Work out the finished part from the listing and answer in its coordinate system (mm). A direction names the side the tool comes from. Give positions to 0.01 mm unless a question says otherwise; leave off trailing zeros. Loops run counter-clockwise (first coordinate to the right, second up) from the corner with the lowest first, then second, coordinate; pieces in that order, holes last. Notation, with made-up numbers: M 1,19 L 39,19 A20 ccw 39,47 Z; hole C 7,27.5 d2. An arc over 180 degrees is marked long. Write item = value, one per line. Start each with the question number.
1. Section B-B on z = -53 is taken. Determine the outline of the cut face in (x, y).
2. Section A-A on y = -85.5 is taken. Determine the outline of the cut face in (x, z), plus the area to 3 significant figures.
3. For faces 1 (the face through (51.969, -98.243, -40.28)), 2 (the face through (57, -63, -2)), 3 (the face through (57, -66.314, -40)), determine the directions among +Z, -Z, +X, -X, +Y, -Y from which every point of the face is accessible in a straight line to the end or side of a thin tool.
4. Consider L1, parallel to X at y = -79, z = -40.5; L2, parallel to Y at x = 60.5, z = -22.5; L3, parallel to Z at x = 56.5, y = -108. Determine where each line is inside the solid, lowest interval first. Write a range as [from, to].
5. Section D-D on z = -16 is taken. Determine the outline of the cut face in (x, y).
6. Flat-ended cylindrical pins translate along their axes: pin 1 Ø6 at (y, z) = (-64, -52.5) entering from +X; pin 2 Ø14 at (y, z) = (-78.5, -50) entering from +X; pin 3 Ø6.5 at (x, z) = (57.5, -47) entering from +Y. Find the tip coordinate at first contact, or state that the pin passes through.
7. Section C-C on x = 60 is taken. Determine the outline of the cut face in (y, z).
```python
from build123d import *

# Parameters (mm, degrees)
SKETCH1_W           = 30
SKETCH1_H           = 70
BOSS_EXTRUDE1_DEPTH = 20
FILLET1_R           = 10
FILLET2_R           = 2
CHAMFER1_SIZE       = 5
CHAMFER1_SIZE2      = 10
FILLET3_R           = 5
SKETCH2_W           = 12
SKETCH2_H           = 32.5
BOSS_EXTRUDE2_DEPTH = 45
FILLET4_R           = 5
SKETCH3_R           = 7
CUT_EXTRUDE1_DEPTH  = 2
FILLET5_R           = 2


with BuildPart() as part:
    # Sketch1 → Boss-Extrude1 (new body)
    with BuildSketch(Plane.XY):
        with Locations((57.367254616, -81.313756287)):
            Rectangle(SKETCH1_W, SKETCH1_H)
    extrude(amount=-BOSS_EXTRUDE1_DEPTH)

    # Fillet1
    fillet1_edges = [part.edges().sort_by_distance(p)[0] for p in [
        (42.367254616, -46.313756287, -10),
        (72.367254616, -46.313756287, -10),
        (72.367254616, -116.313756287, -10),
        (42.367254616, -116.313756287, -10),
    ]]
    fillet(fillet1_edges, radius=FILLET1_R)

    # Fillet2
    fillet2_edges = [part.edges().sort_by_distance(p)[0] for p in [
        (57.367254616, -46.313756287, 0),
        (42.367254616, -81.313756287, 0),
        (57.367254616, -116.313756287, 0),
        (72.367254616, -81.313756287, 0),
        (69.438322428, -113.384824099, 0),
        (45.296186805, -113.384824099, 0),
        (69.438322428, -49.242688475, 0),
        (45.296186805, -49.242688475, 0),
    ]]
    fillet(fillet2_edges, radius=FILLET2_R)

    # Chamfer1
    chamfer1_edges = [part.edges().sort_by_distance(p)[0] for p in [
        (57.367254616, -46.313756287, -20),
        (42.367254616, -81.313756287, -20),
        (72.367254616, -81.313756287, -20),
        (57.367254616, -116.313756287, -20),
        (69.438322428, -113.384824099, -20),
        (45.296186805, -113.384824099, -20),
        (69.438322428, -49.242688475, -20),
        (45.296186805, -49.242688475, -20),
    ]]
    chamfer1_side = [part.faces().sort_by_distance(p)[0] for p in [
        (57.367254616, -81.313756287, -20),
    ]]
    chamfer(chamfer1_edges, length=CHAMFER1_SIZE, length2=CHAMFER1_SIZE2, reference=chamfer1_side[0])

    # Fillet3
    fillet3_edges = [part.edges().sort_by_distance(p)[0] for p in [
        (42.367254616, -81.313756287, -10),
        (67.367254616, -81.313756287, -20),
        (65.902788522, -52.778222381, -20),
        (65.902788522, -109.849290193, -20),
        (57.367254616, -51.313756287, -20),
        (57.367254616, -111.313756287, -20),
        (48.83172071, -52.778222381, -20),
        (48.83172071, -109.849290193, -20),
        (47.367254616, -81.313756287, -20),
        (45.296186805, -113.384824099, -10),
        (45.296186805, -49.242688475, -10),
        (57.367254616, -116.313756287, -10),
        (57.367254616, -46.313756287, -10),
        (69.438322428, -113.384824099, -10),
        (69.438322428, -49.242688475, -10),
        (72.367254616, -81.313756287, -10),
    ]]
    fillet(fillet3_edges, radius=FILLET3_R)

    # Sketch2 → Boss-Extrude2 (add)
    with BuildSketch(Plane(origin=(0, 0, -20), x_dir=(-1, 0, 0), z_dir=(0, 0, -1))):
        with Locations((-57.367254616, -82.563756287)):
            Rectangle(SKETCH2_W, SKETCH2_H)
    extrude(amount=BOSS_EXTRUDE2_DEPTH)

    # Fillet4
    fillet4_edges = [part.edges().sort_by_distance(p)[0] for p in [
        (57.367254616, -98.813756287, -65),
        (57.367254616, -66.313756287, -65),
    ]]
    fillet(fillet4_edges, radius=FILLET4_R)

    # Sketch3 → Cut-Extrude1 (cut)
    with BuildSketch(Plane.XY):
        with Locations((57.367254616, -63.313756287)):
            Circle(SKETCH3_R)
    extrude(amount=-CUT_EXTRUDE1_DEPTH, mode=Mode.SUBTRACT)

    # Fillet5
    fillet5_edges = [part.edges().sort_by_distance(p)[0] for p in [
        (63.367254616, -82.563756287, -65),
        (51.367254616, -82.563756287, -65),
        (63.367254616, -98.813756287, -40),
        (63.367254616, -66.313756287, -40),
        (63.367254616, -97.349290193, -63.535533906),
        (63.367254616, -67.778222381, -63.535533906),
        (51.367254616, -66.313756287, -40),
        (51.367254616, -98.813756287, -40),
        (51.367254616, -97.349290193, -63.535533906),
        (51.367254616, -67.778222381, -63.535533906),
    ]]
    fillet(fillet5_edges, radius=FILLET5_R)


solid = part.part
```
Verdict:
q1.outline = M 51.37,-96.81 A2 ccw 53.37,-98.81 L 61.37,-98.81 A2 ccw 63.37,-96.81 L 63.37,-68.31 A2 ccw 61.37,-66.31 L 53.37,-66.31 A2 ccw 51.37,-68.31 Z
q2.outline = M 42.37,-8.82 A5 ccw 42.9,-11.06 L 45.99,-17.24 A5 ccw 50.46,-20 L 51.37,-20 L 51.37,-63 A2 ccw 53.37,-65 L 61.37,-65 A2 ccw 63.37,-63 L 63.37,-20 L 64.28,-20 A5 ccw 68.75,-17.24 L 71.84,-11.06 A5 ccw 72.37,-8.82 L 72.37,-2 A2 ccw 70.37,0 L 44.37,0 A2 ccw 42.37,-2 Z
q2.area = 1,080 mm2
q3.face_1 = -Z, -X, -Y
q3.face_2 = +Z
q3.face_3 = -Z, +X, -X, +Y
q4.L1 = [51.37, 63.37]
q4.L2 = [-98.81, -66.31]
q4.L3 = [-20, 0]
q5.outline = M 45.37,-106.31 A7 ccw 52.37,-113.31 L 62.37,-113.31 A7 ccw 69.37,-106.31 L 69.37,-56.31 A7 ccw 62.37,-49.31 L 52.37,-49.31 A7 ccw 45.37,-56.31 Z
q6.pin_1 = 62.88
q6.pin_2 = 63.37
q6.pin_3 = -66.31
q7.outline = M -116.31,-8.82 A5 ccw -115.79,-11.06 L -112.7,-17.24 A5 ccw -108.22,-20 L -98.81,-20 L -98.81,-60 A5 ccw -93.81,-65 L -71.31,-65 A5 ccw -66.31,-60 L -66.31,-20 L -54.4,-20 A5 ccw -49.93,-17.24 L -46.84,-11.06 A5 ccw -46.31,-8.82 L -46.31,-2 A2 ccw -48.31,0 L -56.83,0 L -56.83,-2 L -69.8,-2 L -69.8,0 L -114.31,0 A2 ccw -116.31,-2 Z
